Check sheet for the modelled part. Datum: model origin and axes. Units: mm. A direction names the side the tool comes from. Round coordinates to 2 decimals unless told otherwise and drop trailing zeros. Loops run counter-clockwise (first coordinate to the right, second up) from the corner with the lowest first, then second, coordinate; pieces in that order, holes last. Notation, with made-up numbers: (31.5, 44.5) -> (58.5, 44.5) arc R17 cw to (58.5, 69.5) -> close; hole circle Ø10 at (89, -1). An arc over 180 degrees is marked (long way). Return JSON: item names as keys, results as strings.
from build123d import *
from build123d.topology import SkipClean

# Parameters (mm, degrees)
BOSS_EXTRUDE1_DEPTH           = 3
BOSS_EXTRUDE2_START           = -0.5
SKETCH1_3_R                   = 11
BOSS_EXTRUDE2_DEPTH           = 0.5
SKETCH2_R                     = 4.1
SKETCH2_R_2                   = 1.1
CUT_EXTRUDE1_DEPTH            = 3.5
SKETCH2_3_R                   = 2
CUT_EXTRUDE2_DEPTH            = 2.5
CIRPATTERN2_COUNT             = 4
SKETCH1_6_W                   = 11
SKETCH1_6_H                   = 5.42
BOSS_EXTRUDE3_DEPTH           = 6
SKETCH3_R                     = 1.1
CUT_EXTRUDE3_DEPTH            = 9
SKETCH3_3_R                   = 2
SKETCH3_3_R_2                 = 1.1
CUT_EXTRUDE4_DEPTH            = 8
BODY_MOVE_COPY1_START         = -3
BODY_MOVE_COPY1_OUTLINE_R     = 2
BODY_MOVE_COPY1_OUTLINE_R_2   = 4.1
BODY_MOVE_COPY1_DEPTH         = 3
BODY_MOVE_COPY1_START_2       = 3
BODY_MOVE_COPY1_2_OUTLINE_W   = 22
BODY_MOVE_COPY1_2_OUTLINE_H   = 5.42
BODY_MOVE_COPY1_2_OUTLINE_R   = 2
BODY_MOVE_COPY1_2_DEPTH       = 3
BODY_MOVE_COPY1_START_3       = 5
BODY_MOVE_COPY1_3_OUTLINE_R   = 2
BODY_MOVE_COPY1_3_OUTLINE_R_2 = 1.1
BODY_MOVE_COPY1_3_DEPTH       = 1
BODY_MOVE_COPY1_START_4       = 0.5
BODY_MOVE_COPY1_4_OUTLINE_R   = 2
BODY_MOVE_COPY1_4_OUTLINE_R_2 = 4.1
BODY_MOVE_COPY1_4_DEPTH       = 2.5
BODY_MOVE_COPY1_START_5       = -6
BODY_MOVE_COPY1_5_OUTLINE_W   = 22
BODY_MOVE_COPY1_5_OUTLINE_H   = 5.42
BODY_MOVE_COPY1_5_OUTLINE_R   = 1.1
BODY_MOVE_COPY1_5_DEPTH       = 3
BODY_MOVE_COPY1_6_DEPTH       = 0.5


# Read off the part's stored shape, not the designer's step: Body-Move/Copy1
with BuildPart() as part:
    # Sketch1 → Boss-Extrude1 (new body)
    with BuildSketch(Plane.XY):
        with BuildLine():
            Line((-11, 29.235), (-11, -29.235))
            Line((-11, -29.235), (11, -29.235))
            Line((11, -29.235), (11, 29.235))
            ThreePointArc((11, 29.235), (0, 40.235), (-11, 29.235))
        make_face()
        with BuildLine():
            Line((5, -22.815), (-5, -22.815))
            Line((-5, -22.815), (-5, 18.878842411))
            ThreePointArc((-5, 18.878842411), (0, 17.735), (5, 18.878842411))
            Line((5, 18.878842411), (5, -22.815))
        make_face(mode=Mode.SUBTRACT)
    extrude(amount=BOSS_EXTRUDE1_DEPTH)

    # Sketch1<3> → Boss-Extrude2 (add)
    with BuildSketch(Plane.XY.offset(BOSS_EXTRUDE2_START)):
        with Locations((0, 29.235)):
            Circle(SKETCH1_3_R)
    extrude(amount=BOSS_EXTRUDE2_DEPTH)

    # Sketch2 → Cut-Extrude1 (cut)
    with BuildSketch(Plane.XY.offset(3)):
        with Locations((0, 29.235)):
            Circle(SKETCH2_R)
        with Locations((5.656854249, 34.891854249)):
            Circle(SKETCH2_R_2)
    cut_extrude1 = extrude(amount=-CUT_EXTRUDE1_DEPTH, mode=Mode.SUBTRACT)

    # Sketch2<3> → Cut-Extrude2 (cut)
    with BuildSketch(Plane.XY.offset(3)):
        with Locations((5.656854249, 34.891854249)):
            Circle(SKETCH2_3_R)
    cut_extrude2 = extrude(amount=-CUT_EXTRUDE2_DEPTH, mode=Mode.SUBTRACT)

    # CirPattern2: Cut-Extrude1, Cut-Extrude2 ×4 about axis
    cirpattern2_axis = Axis((0, 29.235, 0), (0, 0, 1))
    add([cut_extrude1.rotate(cirpattern2_axis, i * 360 / CIRPATTERN2_COUNT) for i in range(1, CIRPATTERN2_COUNT)], mode=Mode.SUBTRACT)
    add([cut_extrude2.rotate(cirpattern2_axis, i * 360 / CIRPATTERN2_COUNT) for i in range(1, CIRPATTERN2_COUNT)], mode=Mode.SUBTRACT)

    # Sketch1<6> → Boss-Extrude3 (add)
    with BuildSketch(Plane.XY):
        with Locations((-5.5, -26.525)):
            Rectangle(SKETCH1_6_W, SKETCH1_6_H)
        with Locations((5.5, -26.525)):
            Rectangle(SKETCH1_6_W, SKETCH1_6_H)
    extrude(amount=-BOSS_EXTRUDE3_DEPTH)

    # Sketch3 → Cut-Extrude3 (cut)
    with BuildSketch(Plane.XY.offset(3)):
        with Locations((-8.5, -26.62018786)):
            Circle(SKETCH3_R)
        with Locations((8.5, -26.62018786)):
            Circle(SKETCH3_R)
    extrude(amount=-CUT_EXTRUDE3_DEPTH, mode=Mode.SUBTRACT)

    # Sketch3<3> → Cut-Extrude4 (cut)
    # profile 1 of 2: a face of its own
    with BuildSketch(Plane.XY.offset(3)):
        with Locations((-8.5, -26.62018786)):
            Circle(SKETCH3_3_R)
        with Locations((-8.5, -26.62018786)):
            Circle(SKETCH3_3_R_2, mode=Mode.SUBTRACT)
    # profile 2 of 2: a face of its own
    with BuildSketch(Plane.XY.offset(3)):
        with Locations((8.5, -26.62018786)):
            Circle(SKETCH3_3_R)
        with Locations((8.5, -26.62018786)):
            Circle(SKETCH3_3_R_2, mode=Mode.SUBTRACT)
    extrude(amount=-CUT_EXTRUDE4_DEPTH, mode=Mode.SUBTRACT)

    # Body-Move/Copy1 outline → Body-Move/Copy1 (add)
    with BuildSketch(Plane.XY.offset(BODY_MOVE_COPY1_START)):
        with BuildLine():
            Line((-11, -23.815), (11, -23.815))
            Line((11, -23.815), (11, 29.235))
            ThreePointArc((11, 29.235), (0, 40.235), (-11, 29.235))
            Line((-11, 29.235), (-11, -23.815))
        make_face()
        with BuildLine():
            Line((5, 18.878842411), (5, -22.815))
            Line((5, -22.815), (-5, -22.815))
            Line((-5, -22.815), (-5, 18.878842411))
            ThreePointArc((-5, 18.878842411), (0, 17.735), (5, 18.878842411))
        make_face(mode=Mode.SUBTRACT)
        with Locations((5.656854249, 34.891854249)):
            Circle(BODY_MOVE_COPY1_OUTLINE_R, mode=Mode.SUBTRACT)
        with Locations((-5.656854249, 23.578145751)):
            Circle(BODY_MOVE_COPY1_OUTLINE_R, mode=Mode.SUBTRACT)
        with Locations((-5.656854249, 34.891854249)):
            Circle(BODY_MOVE_COPY1_OUTLINE_R, mode=Mode.SUBTRACT)
        with Locations((0, 29.235)):
            Circle(BODY_MOVE_COPY1_OUTLINE_R_2, mode=Mode.SUBTRACT)
        with Locations((5.656854249, 23.578145751)):
            Circle(BODY_MOVE_COPY1_OUTLINE_R, mode=Mode.SUBTRACT)
    extrude(amount=BODY_MOVE_COPY1_DEPTH)

    # Body-Move_Copy1 2 outline → Body-Move_Copy1 2 (add)
    with BuildSketch(Plane.XY.offset(BODY_MOVE_COPY1_START_2)):
        with Locations((0, -26.525)):
            Rectangle(BODY_MOVE_COPY1_2_OUTLINE_W, BODY_MOVE_COPY1_2_OUTLINE_H)
        with Locations((-8.5, -26.62018786)):
            Circle(BODY_MOVE_COPY1_2_OUTLINE_R, mode=Mode.SUBTRACT)
        with Locations((8.5, -26.62018786)):
            Circle(BODY_MOVE_COPY1_2_OUTLINE_R, mode=Mode.SUBTRACT)
    extrude(amount=BODY_MOVE_COPY1_2_DEPTH)

    # Body-Move_Copy1 3 outline → Body-Move_Copy1 3 (add)
    # profile 1 of 2: a face of its own
    with BuildSketch(Plane.XY.offset(BODY_MOVE_COPY1_START_3)):
        with Locations((-8.5, -26.62018786)):
            Circle(BODY_MOVE_COPY1_3_OUTLINE_R)
        with Locations((-8.5, -26.62018786)):
            Circle(BODY_MOVE_COPY1_3_OUTLINE_R_2, mode=Mode.SUBTRACT)
    # profile 2 of 2: a face of its own
    with BuildSketch(Plane.XY.offset(BODY_MOVE_COPY1_START_3)):
        with Locations((8.5, -26.62018786)):
            Circle(BODY_MOVE_COPY1_3_OUTLINE_R)
        with Locations((8.5, -26.62018786)):
            Circle(BODY_MOVE_COPY1_3_OUTLINE_R_2, mode=Mode.SUBTRACT)
    extrude(amount=BODY_MOVE_COPY1_3_DEPTH)

    # Body-Move_Copy1 4 outline → Body-Move_Copy1 4 (cut)
    with BuildSketch(Plane.XY.offset(BODY_MOVE_COPY1_START_4)):
        with BuildLine():
            Line((-11, -23.815), (11, -23.815))
            Line((11, -23.815), (11, 29.235))
            ThreePointArc((11, 29.235), (0, 40.235), (-11, 29.235))
            Line((-11, 29.235), (-11, -23.815))
        make_face()
        with BuildLine():
            Line((5, 18.878842411), (5, -22.815))
            Line((5, -22.815), (-5, -22.815))
            Line((-5, -22.815), (-5, 18.878842411))
            ThreePointArc((-5, 18.878842411), (0, 17.735), (5, 18.878842411))
        make_face(mode=Mode.SUBTRACT)
        with Locations((5.656854249, 34.891854249)):
            Circle(BODY_MOVE_COPY1_4_OUTLINE_R, mode=Mode.SUBTRACT)
        with Locations((-5.656854249, 23.578145751)):
            Circle(BODY_MOVE_COPY1_4_OUTLINE_R, mode=Mode.SUBTRACT)
        with Locations((-5.656854249, 34.891854249)):
            Circle(BODY_MOVE_COPY1_4_OUTLINE_R, mode=Mode.SUBTRACT)
        with Locations((0, 29.235)):
            Circle(BODY_MOVE_COPY1_4_OUTLINE_R_2, mode=Mode.SUBTRACT)
        with Locations((5.656854249, 23.578145751)):
            Circle(BODY_MOVE_COPY1_4_OUTLINE_R, mode=Mode.SUBTRACT)
    extrude(amount=BODY_MOVE_COPY1_4_DEPTH, mode=Mode.SUBTRACT)

    # Body-Move_Copy1 5 outline → Body-Move_Copy1 5 (cut)
    with BuildSketch(Plane.XY.offset(BODY_MOVE_COPY1_START_5)):
        with Locations((0, -26.525)):
            Rectangle(BODY_MOVE_COPY1_5_OUTLINE_W, BODY_MOVE_COPY1_5_OUTLINE_H)
        with Locations((-8.5, -26.62018786)):
            Circle(BODY_MOVE_COPY1_5_OUTLINE_R, mode=Mode.SUBTRACT)
        with Locations((8.5, -26.62018786)):
            Circle(BODY_MOVE_COPY1_5_OUTLINE_R, mode=Mode.SUBTRACT)
    extrude(amount=BODY_MOVE_COPY1_5_DEPTH, mode=Mode.SUBTRACT)

    # Body-Move_Copy1 6 outline → Body-Move_Copy1 6 (cut)
    with SkipClean():  # the faces are left unmerged after this step: merging them gives an invalid solid
        with BuildSketch(Plane.XY):
            with BuildLine():
                Line((-11, -23.815), (11, -23.815))
                Line((11, -23.815), (11, 29.235))
                ThreePointArc((11, 29.235), (0, 18.235), (-11, 29.235))
                Line((-11, 29.235), (-11, -23.815))
            make_face()
            with BuildLine():
                Line((5, 18.878842411), (5, -22.815))
                Line((5, -22.815), (-5, -22.815))
                Line((-5, -22.815), (-5, 18.878842411))
                ThreePointArc((-5, 18.878842411), (0, 17.735), (5, 18.878842411))
            make_face(mode=Mode.SUBTRACT)
        extrude(amount=BODY_MOVE_COPY1_6_DEPTH, mode=Mode.SUBTRACT)


solid = part.part
Q1. Tool access check on faces 4 (the flat face through (0, -22.815, -2)), 5 (the flat face through (0, -26, 6)), 6 (the cylindrical face through (-6.09, 32.94, -1.77)). Record the directions out of +Z, -Z, +X, -X, +Y, -Y that give a thin tool (end or side, any length) a straight path to the whole face; none if there is none.
Results list:
{"face 4": "+Z, -Z", "face 5": "+Z, +X, -X, +Y, -Y", "face 6": "-Z"}
Q2. Section check B-B (y = 8.5). Record the boundary of the cut face in (x, z), then the cut area to 3 significant figures.
Results list:
{"outline": "(-11, -3) -> (-5, -3) -> (-5, 0) -> (-11, 0) -> close; (5, -3) -> (11, -3) -> (11, 0) -> (5, 0) -> close", "area": "36.0 mm^2"}
Q3. Draft check along Y on faces 1 (the flat face through (-7, -3, 0)), 2 (the flat face through (0, -29.235, 1)), 3 (the flat face through (-11, -7, -1)). Enter one of: released by +Y, released by -Y, zero draft, split by the parting line, or undercut.
Results list:
{"face 1": "undercut", "face 2": "released by -Y", "face 3": "zero draft"}
Q4. Section check C-C (x = 8.5). Record the boundary of the cut face in (y, z) (3 decimals).
Results list:
{"outline": "(-29.235, -3) -> (-28.62, -3) -> (-28.62, 5) -> (-27.72, 5) -> (-27.72, 6) -> (-29.235, 6) -> close; (-25.52, 5) -> (-24.62, 5) -> (-24.62, -3) -> (36.217, -3) -> (36.217, 0.5) -> (22.253, 0.5) -> (22.253, 0) -> (-23.815, 0) -> (-23.815, 6) -> (-25.52, 6) -> close"}
Q5. Go/stop test with flat-tipped pins: pin 1 (3.5 mm diameter, centred on x = 5.66, y = 23.58, fed in from +Z); pin 2 (3 mm diameter, centred on x = -5.5, y = 34.5, fed in from -Z); pin 3 (3 mm diameter, centred on y = 33, z = -1, fed in from +X). Record where each tip stops, or that it passes through.
Results list:
{"pin 1": "z = 0.5", "pin 2": "z = -0.5", "pin 3": "x = 10.76"}
Q6. Material ranges on line 1 (X direction, y = -20.5, z = -0.25); line 2 (Y direction, x = 0.75, z = -0.75) (3 decimals); line 3 (Y direction, x = -1.5, z = 4.5) (3 decimals), recorded low to high.
Results list:
{"line 1": "-11 to -5, 5 to 11", "line 2": "-29.235 to -22.815, 17.759 to 25.204, 33.266 to 40.209", "line 3": "-29.235 to -23.815"}
Q7. Section check A-A (x = 0). Record the boundary of the cut face in (y, z) (3 decimals).
Results list:
{"outline": "(-29.235, -3) -> (-22.815, -3) -> (-22.815, 0) -> (-23.815, 0) -> (-23.815, 6) -> (-29.235, 6) -> close; (17.735, -3) -> (25.135, -3) -> (25.135, 0.5) -> (18.235, 0.5) -> (18.235, 0) -> (17.735, 0) -> close; (33.335, -3) -> (40.235, -3) -> (40.235, 0.5) -> (33.335, 0.5) -> close"}
Q8. Section check D-D (x = 2.75). Record the boundary of the cut face in (y, z) (3 decimals).
Results list:
{"outline": "(-29.235, -3) -> (-22.815, -3) -> (-22.815, 0) -> (-23.815, 0) -> (-23.815, 6) -> (-29.235, 6) -> close; (18.069, -3) -> (26.194, -3) -> (26.194, 0.5) -> (18.584, 0.5) -> (18.584, 0) -> (18.069, 0) -> close; (32.276, -3) -> (39.886, -3) -> (39.886, 0.5) -> (32.276, 0.5) -> close"}
